Could you check a few things on this model? Use its own coordinates, in mm. Coordinates: 2 decimals unless noted, no trailing zeros. Order: outer loops, then holes, each group sorted by start corner. A loop starts at its lowest first (then second) coordinate and runs counter-clockwise, first axis right, second up. Notation, with made-up numbers: M -36.75,2 L 21.25,2 A25 ccw 21.25,32 Z; hole C -21.5,74.25 d2. An arc over 180 degrees is marked long. Put each result on its own line as item: value. Start each with the question number.
```python
from build123d import *

# Parameters (mm, degrees)
F1_DEPTH = 6
F3_DEPTH = 6.001
F4_R     = 2.75
F5_DEPTH = 40.001
F6_R     = 2.99999
F7_DEPTH = 6.001


# Not quite as in the source:
# - a fillet or chamfer is up to 0.001 mm smaller than in the source, because OpenCascade refuses the exact size


with BuildPart() as f1:
    # F0 (on Top) → F1 (new body)
    with BuildSketch(Plane.XY):
        with BuildLine():
            Line((-8.5178157315, -13.6271222085), (-38.8432986429, -13.6271222085))
            Line((-38.8432986429, -13.6271222085), (-38.8432986429, -19.6271222085))
            Line((-38.8432986429, -19.6271222085), (-8.5178157315, -19.6271222085))
            ThreePointArc((-8.5178157315, -19.6271222085), (-11.5178157315, -16.6271222085), (-8.5178157315, -13.6271222085))
        make_face()
        with BuildLine():
            Line((1.1567013571, -13.6271222085), (-8.5178157315, -13.6271222085))
            ThreePointArc((-8.5178157315, -13.6271222085), (-6.3964953879, -14.5058018649), (-5.5178157315, -16.6271222085))
            ThreePointArc((-5.5178157315, -16.6271222085), (-6.3964953879, -18.748442552), (-8.5178157315, -19.6271222085))
            Line((-8.5178157315, -19.6271222085), (1.1567013571, -19.6271222085))
            Line((1.1567013571, -19.6271222085), (1.1567013571, -13.6271222085))
        make_face()
        with BuildLine():
            ThreePointArc((-5.5178157315, -16.6271222085), (-6.3964953879, -14.5058018649), (-8.5178157315, -13.6271222085))
            ThreePointArc((-8.5178157315, -13.6271222085), (-11.5178157315, -16.6271222085), (-8.5178157315, -19.6271222085))
            ThreePointArc((-8.5178157315, -19.6271222085), (-6.3964953879, -18.748442552), (-5.5178157315, -16.6271222085))
        make_face()
    extrude(amount=F1_DEPTH)

    # F2 (on face) → F3 (cut, through all)
    with BuildSketch(Plane.XZ.offset(19.6271222085)):
        Polygon((1.1567013571, 6), (-4.8432986429, 6), (1.1567013571, 0), align=None)
    extrude(amount=-F3_DEPTH, mode=Mode.SUBTRACT)

    # F4 (on face) → F5 (cut, through all)
    with BuildSketch(Plane(origin=(-38.8432986429, 0, 0), x_dir=(0, -1, 0), z_dir=(-1, 0, 0))):
        with Locations((16.6271222085, 3)):
            Circle(F4_R)
    extrude(amount=-F5_DEPTH, mode=Mode.SUBTRACT)

    # F6 (radius 3 in the source; OpenCascade refuses exactly that, so slightly less here)
    f6_edges = [f1.edges().sort_by_distance(p)[0] for p in [
        (-21.843299, -19.627122, 6),
        (-21.843299, -13.627122, 6),
        (-18.843299, -13.627122, 0),
        (-18.843299, -19.627122, 0),
    ]]
    fillet(f6_edges, radius=F6_R)

    # F2 (on face) → F7 (cut, through all)
    with BuildSketch(Plane.XZ.offset(19.6271222085)):
        Polygon((-38.8432986429, 0), (-32.8432986429, 6), (-38.8432986429, 6), align=None)
    extrude(amount=-F7_DEPTH, mode=Mode.SUBTRACT)


solid = f1.part
```
Item 1: If we section it at C-C on z = 4: Write out the boundary of the cut face in (x, y), then the cut area to 3 significant figures.
Item 2: If we mould it in two halves opening along Z, with no side actions, what happens to faces 1 (the cylindrical face through (-19.081, -14.483, 5.098)), 2 (the cylindrical face through (-19.087, -16.031, 0.315)), 3 (the cylindrical face through (-19.123, -14.483, 0.902))? For each: released by +Z, released by -Z, zero draft, split by the parting line, or undercut.
Item 3: For pin 1 Ø3.5 at (y, z) = (-16.63, 3) entering from -X; pin 2 Ø1.5 at (x, z) = (-6.5, 4) entering from +Y; pin 3 Ø1.5 at (y, z) = (-17.5, 1) entering from -X; pin 4 Ø1 at (x, y) = (-19, -18) entering from -Z, each with a flat end and sliding along its axis, tell me the tip position at first contact or that it passes through.
Item 4: I need wall thicknesses on probe 1 along Y at (x, z) = (-17, 3); probe 2 along Z at (x, y) = (-12.5, -16.5); probe 3 along Z at (x, y) = (-37, -16.75). Which ranges of each line are inside material? Lowest first, please.
Item 5: If we section it at A-A on y = -18.5: Write out the boundary of the cut face in (x, z), then the cut area to 3 significant figures.
Geometry check:
1. outline: M -34.84,-19.46 L -2.84,-19.46 L -2.84,-19.19 L -34.84,-19.19 Z; M -34.84,-14.07 L -2.84,-14.07 L -2.84,-13.8 L -34.84,-13.8 Z
1. area: 17.1 mm²
2. face 1: released by +Z
2. face 2: undercut
2. face 3: released by -Z
3. pin 1: passes through
3. pin 2: stops at y = -13.64
3. pin 3: stops at x = -38.59
3. pin 4: stops at z = 0.13
4. probe 1: y = -19.63 to -19.38, -13.88 to -13.63
4. probe 2: z = 0 to 0.25, 5.75 to 6
4. probe 3: z = 0 to 0.25
5. outline: M -38.19,0.66 L 0.5,0.66 L 0.17,0.99 L -37.86,0.99 Z; M -33.83,5.01 L -3.86,5.01 L -4.19,5.34 L -33.5,5.34 Z
5. area: 22.4 mm²
